```python
from build123d import *

# Parameters (mm, degrees)
ESQUISSE1_R             = 2.5
BOSS_EXTRU_1_DEPTH      = 186
ENL_V_MAT_EXTRU_1_DEPTH = 1


with BuildPart() as part:
    # Esquisse1 → Boss.-Extru.1 (new body)
    with BuildSketch(Plane.XY):
        with Locations(Location((0, 0, 0), (0, 0, 180))):
            Circle(ESQUISSE1_R)
    extrude(amount=BOSS_EXTRU_1_DEPTH)

    # Esquisse2 → Enlèv. mat.-Extru.1 (cut)
    with BuildSketch(Plane(origin=(0, 0, 0), x_dir=(-1, 0, 0), z_dir=(0, 0, -1))):
        with BuildLine():
            Line((-0.5, 2.449489743), (-0.5, -2.449489743))
            ThreePointArc((-0.5, -2.449489743), (0, -2.5), (0.5, -2.449489743))
            Line((0.5, -2.449489743), (0.5, 2.449489743))
            ThreePointArc((0.5, 2.449489743), (0, 2.5), (-0.5, 2.449489743))
        make_face()
    extrude(amount=-ENL_V_MAT_EXTRU_1_DEPTH, mode=Mode.SUBTRACT)


solid = part.part
```
Geometry: final body of the model. Coordinates: model frame, mm. Give positions to 0.01 mm unless a question says otherwise; leave off trailing zeros. Loops run counter-clockwise (first coordinate to the right, second up) from the corner with the lowest first, then second, coordinate; pieces in that order, holes last. Notation, with made-up numbers: (44.25, 44) -> (79.25, 44) arc R17 cw to (79.25, 71) -> close; hole circle Ø8 at (36, 78.25). An arc over 180 degrees is marked (long way). Use one line per item in the form item = value.
Item 1: Section query B-B on y = 1.2. Output: boundary loops of the cut face in (x, z).
A:
outline = (-2.19, 0) -> (-0.5, 0) -> (-0.5, 1) -> (0.5, 1) -> (0.5, 0) -> (2.19, 0) -> (2.19, 186) -> (-2.19, 186) -> close
Item 2: Section query A-A on z = 114.5. Output: boundary loops of the cut face in (x, y), and give its area (3 significant figures).
A:
outline = circle Ø5 at (0, 0)
area = 19.6 mm^2
Item 3: Section query C-C on x = -1.6. Output: boundary loops of the cut face in (y, z), and give its area (3 significant figures).
A:
outline = (-1.92, 0) -> (1.92, 0) -> (1.92, 186) -> (-1.92, 186) -> close
area = 715 mm^2
Item 4: Pin query (flat end, axial travel): P1, Ø0.5, axis at y = 1, z = 0.5, coming from the -X side; P2, Ø1.1, axis at y = -1, z = 0.5, coming from the +X side; P3, Ø2, axis at y = 1.5, z = 136.5, coming from the +X side. Return the tip coordinate at first contact, or that it passes through.
A:
P1 = -2.38
P2 = 2.46
P3 = 2.45
Item 5: Line query: probe 1 along Y at (x, z) = (0.1, 43); probe 2 along X at (y, z) = (-0.65, 25). Output: solid intervals per line, ascending.
A:
probe_1 = -2.5 to 2.5
probe_2 = -2.41 to 2.41
